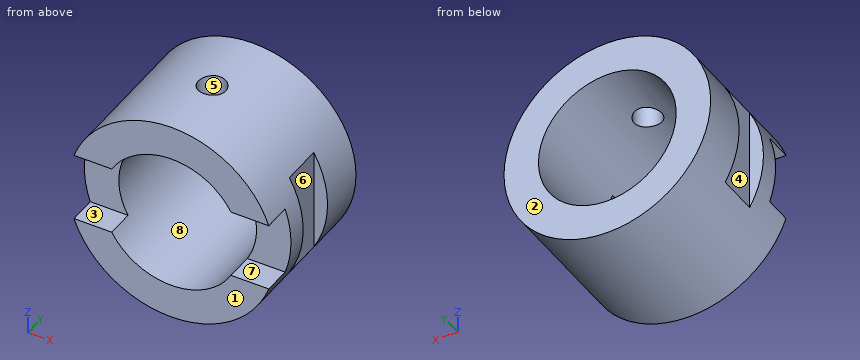
```python
from build123d import *

# Parameters (mm, degrees)
F0_R     = 37.5
F0_R_2   = 25
F1_DEPTH = 25
F2_R     = 5
F3_DEPTH = 37.501
F2_W     = 5
F2_H     = 15
F4_DEPTH = 37.5
F2_W_2   = 75
F2_H_2   = 10
F5_DEPTH = 12.5


with BuildPart() as f1:
    # F0 (on Front) → F1 (new body, symmetric)
    with BuildSketch(Plane.XZ):
        Circle(F0_R)
        Circle(F0_R_2, mode=Mode.SUBTRACT)
    extrude(amount=F1_DEPTH, both=True)

    # F2 (on Top) → F3 (cut, through all)
    with BuildSketch(Plane.XY):
        Circle(F2_R)
    extrude(amount=F3_DEPTH, mode=Mode.SUBTRACT)

    # F2 (on Top) → F4 (cut, symmetric)
    with BuildSketch(Plane.XY):
        with Locations((-35, 0)):
            Rectangle(F2_W, F2_H)
        with Locations((35, 0)):
            Rectangle(F2_W, F2_H)
    extrude(amount=F4_DEPTH, both=True, mode=Mode.SUBTRACT)

    # F2 (on Top) → F5 (cut, symmetric)
    with BuildSketch(Plane.XY):
        with Locations((0, -20)):
            Rectangle(F2_W_2, F2_H_2)
    extrude(amount=F5_DEPTH, both=True, mode=Mode.SUBTRACT)


solid = f1.part
```
Geometry check sheet. Reference: the model listing, model coordinates, mm. Face numbers are marked on the shaded views. A direction names the side the tool comes from. Coordinates: 2 decimals unless noted, no trailing zeros. Loops run counter-clockwise (first coordinate to the right, second up) from the corner with the lowest first, then second, coordinate; pieces in that order, holes last.
Item 1: Sectioned sample at A-A, the plane x = 0. Record the boundary of the cut face in (y, z).
Item 2: Release check for a two-part mould opening along X. For the marked faces 6, 7 and 8 record: released by +X, released by -X, zero draft, split by the parting line, or undercut.
Item 3: Access from +Z, -Z, +X, -X, +Y, -Y to the whole of each face (thin tool, end or side, straight path). Record for the marked faces 1, 2, 3, 4 and 5.
Item 4: Go/stop test with flat-tipped pins: pin 1 Ø1.5 at (x, y) = (-27, 16.5) entering from +Z; pin 2 Ø16.5 at (y, z) = (-2.5, 7) entering from +X; pin 3 Ø2 at (y, z) = (0.5, 14.5) entering from +X. Record where each tip stops, or that it passes through.
Item 5: Sectioned sample at B-B, the plane z = 0. Record the boundary of the cut face in (x, y).
Item 6: Thickness scan on line 1 (Y direction, x = 0, z = 30); line 2 (X direction, y = 15, z = 0); line 3 (Z direction, x = 1, y = 9). Record the ranges inside material, lowest first.
Item 7: Sectioned sample at C-C, the plane y = -18.5. Record the boundary of the cut face in (x, z), then the cut area to 3 significant figures.
Item 8: Sectioned sample at D-D, the plane x = 30. Record the boundary of the cut face in (y, z).
Check result:
1. outline: (-25, -37.5) - (25, -37.5) - (25, -25) - (-25, -25) - close; (-25, 25) - (-5, 25) - (-5, 37.5) - (-25, 37.5) - close; (5, 25) - (25, 25) - (25, 37.5) - (5, 37.5) - close
2. face 6: released by +X
2. face 7: zero draft
2. face 8: undercut
3. face 1: +Z, -Z, +X, -X, -Y
3. face 2: +Z, -Z, +X, -X, +Y
3. face 3: +X, -X, -Y
3. face 4: +Z, -Z, -X
3. face 5: +Z
4. pin 1: stops at z = 26.78
4. pin 2: stops at x = 37.5
4. pin 3: stops at x = 32.5
5. outline: (-37.5, -15) - (-25, -15) - (-25, 25) - (-37.5, 25) - (-37.5, 7.5) - (-32.5, 7.5) - (-32.5, -7.5) - (-37.5, -7.5) - close; (25, -15) - (37.5, -15) - (37.5, -7.5) - (32.5, -7.5) - (32.5, 7.5) - (37.5, 7.5) - (37.5, 25) - (25, 25) - close
6. line 1: y = -25 to -5, 5 to 25
6. line 2: x = -37.5 to -25, 25 to 37.5
6. line 3: z = -37.49 to -24.98, 24.98 to 37.49
7. outline: (-35.36, -12.5) arc R37.5 ccw to (35.36, -12.5) - (21.65, -12.5) arc R25 cw to (-21.65, -12.5) - close; (-35.36, 12.5) - (-21.65, 12.5) arc R25 cw to (21.65, 12.5) - (35.36, 12.5) arc R37.5 ccw to start
7. area: 1,810 mm2
8. outline: (-25, -22.5) - (25, -22.5) - (25, 22.5) - (-25, 22.5) - (-25, 12.5) - (-15, 12.5) - (-15, -12.5) - (-25, -12.5) - close
